Geometry: final body of the model. Coordinates: model frame, mm. Face numbers are marked on the shaded views. A direction names the side the tool comes from. Give positions to 0.01 mm unless a question says otherwise; leave off trailing zeros. Order: outer loops, then holes, each group sorted by start corner. A loop starts at its lowest first (then second) coordinate and runs counter-clockwise, first axis right, second up. Notation, with made-up numbers: M 18,-7 L 40,-7 A26 cw 40,17 Z; hole C 83.5,42 d8. An arc over 180 degrees is marked long. One line per item, written item: value. Start each with the question number.
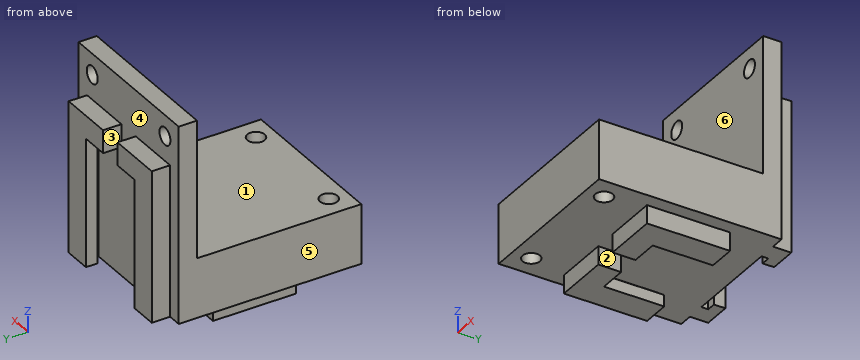
```python
from build123d import *

# Parameters (mm, degrees)
SKETCH1_W               = 29
SKETCH1_H               = 15
BOSS_EXTRUDE1_DEPTH     = 8
SKETCH2_W               = 17
SKETCH2_H               = 2.5
SKETCH2_W_2             = 21
SKETCH2_H_2             = 2
CUT_EXTRUDE1_DEPTH      = 1
CUT_EXTRUDE1_DEPTH_BACK = 16
SKETCH4_W               = 5
SKETCH4_H               = 3.5
BOSS_EXTRUDE2_DEPTH     = 5
SKETCH5_W               = 35
SKETCH5_H               = 30
BOSS_EXTRUDE3_DEPTH     = 4
SKETCH6_R               = 1.905
CUT_EXTRUDE2_DEPTH      = 1
CUT_EXTRUDE2_DEPTH_BACK = 9
SKETCH9_W               = 35
SKETCH9_H               = 39.85
BOSS_EXTRUDE4_DEPTH     = 13
SKETCH10_R              = 1.905
CUT_EXTRUDE4_DEPTH      = 13
SKETCH11_W              = 29
SKETCH11_H              = 13.15
BOSS_EXTRUDE5_DEPTH     = 4
SKETCH12_W              = 17
SKETCH12_H              = 2.5
CUT_EXTRUDE5_DEPTH      = 31.5
SKETCH13_W              = 12
SKETCH13_H              = 4
BOSS_EXTRUDE6_DEPTH     = 5
BOSS_EXTRUDE7_DEPTH     = 13


with BuildPart() as part:
    # Sketch1 → Boss-Extrude1 (new body)
    with BuildSketch(Plane(origin=(0, 0, 0), x_dir=(1, 0, 0), z_dir=(0, 1, 0))):
        with Locations((14.5, 7.5)):
            Rectangle(SKETCH1_W, SKETCH1_H)
    extrude(amount=BOSS_EXTRUDE1_DEPTH)

    # Sketch2 → Cut-Extrude1 (cut, two sides)
    with BuildSketch(Plane.XY) as cut_extrude1_sk:
        with Locations((14.5, 6.75)):
            Rectangle(SKETCH2_W, SKETCH2_H)
        with Locations((14.5, 4.5)):
            Rectangle(SKETCH2_W_2, SKETCH2_H_2)
    extrude(amount=CUT_EXTRUDE1_DEPTH, mode=Mode.SUBTRACT)
    extrude(cut_extrude1_sk.sketch, amount=-CUT_EXTRUDE1_DEPTH_BACK, mode=Mode.SUBTRACT)

    # Sketch4 → Boss-Extrude2 (add)
    with BuildSketch(Plane.XY):
        with Locations((14.5, 1.75)):
            Rectangle(SKETCH4_W, SKETCH4_H)
        Polygon((17, 3.5), (17, 0), (29, 0), (29, 8), (23, 8), (23, 5.5), (25, 5.5), (25, 3.5), align=None)
        Polygon((6, 8), (0, 8), (0, 0), (12, 0), (12, 3.5), (4, 3.5), (4, 5.5), (6, 5.5), align=None)
        Polygon((12, 8), (6, 8), (6, 5.5), (4, 5.5), (4, 3.5), (12, 3.5), align=None)
        Polygon((23, 8), (17, 8), (17, 3.5), (25, 3.5), (25, 5.5), (23, 5.5), align=None)
    extrude(amount=BOSS_EXTRUDE2_DEPTH)

    # Sketch5 → Boss-Extrude3 (add)
    with BuildSketch(Plane(origin=(0, 0, 0), x_dir=(-1, 0, 0), z_dir=(0, -1, 0))):
        with Locations((-14.5, 0)):
            Rectangle(SKETCH5_W, SKETCH5_H)
    extrude(amount=-BOSS_EXTRUDE3_DEPTH)

    # Sketch6 → Cut-Extrude2 (cut, two sides)
    with BuildSketch(Plane(origin=(0, 0, 0), x_dir=(-1, 0, 0), z_dir=(0, -1, 0))) as cut_extrude2_sk:
        with Locations((-27.2, -10.4)):
            Circle(SKETCH6_R)
        with Locations((-1.8, -10.4)):
            Circle(SKETCH6_R)
    extrude(amount=CUT_EXTRUDE2_DEPTH, mode=Mode.SUBTRACT)
    extrude(cut_extrude2_sk.sketch, amount=-CUT_EXTRUDE2_DEPTH_BACK, mode=Mode.SUBTRACT)

    # Sketch9 → Boss-Extrude4 (add)
    with BuildSketch(Plane(origin=(0, 0, -15), x_dir=(-1, 0, 0), z_dir=(0, 0, -1))):
        with Locations((-14.5, -15.925)):
            Rectangle(SKETCH9_W, SKETCH9_H)
    extrude(amount=BOSS_EXTRUDE4_DEPTH)

    # Sketch10 → Cut-Extrude4 (cut)
    with BuildSketch(Plane.XY.offset(-15)):
        with Locations((1.8, -31.75)):
            Circle(SKETCH10_R)
        with Locations((27.2, -31.75)):
            Circle(SKETCH10_R)
    extrude(amount=-CUT_EXTRUDE4_DEPTH, mode=Mode.SUBTRACT)

    # Sketch11 → Boss-Extrude5 (add)
    with BuildSketch(Plane(origin=(0, 0, -28), x_dir=(-1, 0, 0), z_dir=(0, 0, -1))):
        with Locations((-14.5, -11.925)):
            Rectangle(SKETCH11_W, SKETCH11_H)
    extrude(amount=BOSS_EXTRUDE5_DEPTH)

    # Sketch12 → Cut-Extrude5 (cut, through all)
    with BuildSketch(Plane(origin=(0, -5.35, 0), x_dir=(1, 0, 0), z_dir=(0, 1, 0))):
        Polygon((4, 29.5), (4, 28), (25, 28), (25, 29.5), (23, 29.5), (6, 29.5), align=None)
        with Locations((14.5, 30.75)):
            Rectangle(SKETCH12_W, SKETCH12_H)
    extrude(amount=-CUT_EXTRUDE5_DEPTH, mode=Mode.SUBTRACT)

    # Sketch13 → Boss-Extrude6 (add)
    with BuildSketch(Plane(origin=(0, -18.5, 0), x_dir=(-1, 0, 0), z_dir=(0, -1, 0))):
        with Locations((-6, 30)):
            Rectangle(SKETCH13_W, SKETCH13_H)
        with Locations((-23, 30)):
            Rectangle(SKETCH13_W, SKETCH13_H)
    extrude(amount=BOSS_EXTRUDE6_DEPTH)

    # Sketch14 → Boss-Extrude7 (add)
    with BuildSketch(Plane(origin=(0, 0, -15), x_dir=(-1, 0, 0), z_dir=(0, 0, -1))):
        Polygon((0, 4), (0, 8), (-6, 8), (-6, 5.5), (-4, 5.5), (-4, 4), align=None)
        Polygon((-23, 5.5), (-23, 8), (-29, 8), (-29, 4), (-25, 4), (-25, 5.5), align=None)
    extrude(amount=BOSS_EXTRUDE7_DEPTH)


solid = part.part
```
Q1. Section query B-B on z = 10.4. Return loops of the section in (x, y) (3 decimals).
Q2. Set-up query: the marked faces 1, 2 and 3. Return all of +Z, -Z, +X, -X, +Y, -Y with unobstructed straight access to the full face (end or side cutting, diameter ignored); none if empty.
Q3. Section query C-C on y = -31.75. Return loops of the section in (x, z) (3 decimals), and give its area (3 significant figures).
Q4. Section query A-A on x = 27.2. Return loops of the section in (y, z) (3 decimals).
Q5. Mould query, pull axis X, two halves, no side actions, for the marked faces 4, 5 and 6. Classes: +X half, -X half, draft (parallel to the pull), parting line (faces both ways), or undercut.
Q6. Contact query for flat-ended pins moving along their axis: pin 1 (3 mm diameter, centred on x = 12, y = -18, fed in from -Z); pin 2 (2 mm diameter, centred on x = 6.5, z = 8, fed in from -Y); pin 3 (3 mm diameter, centred on x = 27, z = -30.5, fed in from +Y); pin 4 (2 mm diameter, centred on y = 5.5, z = -17.5, fed in from +X). Output: stop coordinate, or through.
Q7. Section query D-D on z = -21.5. Return loops of the section in (x, y) (3 decimals).
Q8. Ray query, line 1 along Z through (x, y) = (1.8, 3) (3 decimals); line 2 along Y through (x, z) = (5, -16.5); line 3 along X through (y, z) = (2.4, 10.4) (3 decimals). Return the intervals inside material, ascending. Write a range as [from, to].
Results below:
1. outline: M -3,0 L -0.105,0 L -0.105,4 L -3,4 Z; M 3.705,0 L 25.295,0 L 25.295,4 L 3.705,4 Z; M 29.105,0 L 32,0 L 32,4 L 29.105,4 Z
2. face 1: +Z, +X, -X, -Y
2. face 2: -Z, +Y, -Y
2. face 3: +Z, -Z, +Y
3. outline: M -3,-28 L -0.105,-28 L -0.105,-15 L -3,-15 Z; M 3.705,-28 L 25.295,-28 L 25.295,-15 L 3.705,-15 Z; M 29.105,-28 L 32,-28 L 32,-15 L 29.105,-15 Z
3. area: 356 mm2
4. outline: M -35.85,-28 L -33.655,-28 L -33.655,-15 L -35.85,-15 Z; M -29.845,-28 L -23.5,-28 L -23.5,-32 L -5.35,-32 L -5.35,-28 L 8,-28 L 8,5 L 4,5 L 4,8.495 L 0,8.495 L 0,-15 L -29.845,-15 Z; M 0,12.305 L 4,12.305 L 4,15 L 0,15 Z
5. face 4: undercut
5. face 5: -X half
5. face 6: draft
6. pin 1: z = -32
6. pin 2: y = 0
6. pin 3: y = -5.35
6. pin 4: x = 29
7. outline: M -3,-35.85 L 32,-35.85 L 32,4 L 29,4 L 29,8 L 23,8 L 23,5.5 L 25,5.5 L 25,4 L 4,4 L 4,5.5 L 6,5.5 L 6,8 L 0,8 L 0,4 L -3,4 Z; hole C 1.8,-31.75 d3.81; hole C 27.2,-31.75 d3.81
8. line 1: [-28, 8.495], [12.305, 15]
8. line 2: [-35.85, 4], [5.5, 8]
8. line 3: [-3, -0.105], [3.705, 25.295], [29.105, 32]
